Autodesk Inventor part; units mm, degrees
ref_plane "YZ Plane" through (0, 0, 0) normal (1, 0, 0) x (0, 1, 0)
ref_plane "XZ Plane" through (0, 0, 0) normal (0, 1, 0) x (-1, 0, 0)
ref_plane "XY Plane" through (0, 0, 0) normal (0, 0, 1) x (1, 0, 0)
sketch "Sketch_1" plane through (0, 0, 0) normal (0, 0, 1) x (1, 0, 0)
  line L0 (55.5, 0) -> (0, 0)
  line L1 (0, 0) -> (0, 2)
  line L2 (0, 2) -> (0.5, 2.5)
  line L3 (0.5, 2.5) -> (55, 2.5)
  line L4 (55, 2.5) -> (55.5, 2)
  line L5 (55.5, 2) -> (55.5, 0)
  line L6 (55.5, 0) -> (0, 0)
revolve "Revolution1" add sketch "Sketch_1" angle 360 about axis through (55.5, 0, 0) along (1, 0, 0)
sketch "Sketch2" plane through (0, 0, 0) normal (-1, 0, 0) x (0, 0, 1)
  point P0 (0, 0)
hole "Hole1" at (0, 0, 0) direction (1, 0, 0) diameter 2.459 depth 8.2901 tip angle 120 countersink diameter 3 countersink angle 90
sketch "Sketch3" plane through (55.5, 0, 0) normal (1, 0, 0) x (0, 0, -1)
  point P0 (0, 0)
hole "Hole2" at (55.5, 0, 0) direction (-1, 0, 0) diameter 2.459 depth 8.2901 tip angle 120 countersink diameter 3 countersink angle 90
properties part number "SETF5-55.5-M3-N3" material "ステンレス鋼 AISI 304"
Verification items for the finished model (mm, model axes). A direction names the side the tool comes from. Round coordinates to 2 decimals unless told otherwise and drop trailing zeros. Write each loop counter-clockwise with the first axis right and the second up, starting at its lowest first coordinate (ties: lowest second). Pieces come first, ordered by that corner, then holes.
1. Section check A-A on x = 39.5. Enter the section's corners in (y, z), plus the area to 3 significant figures.
2. Access from +Z, -Z, +X, -X, +Y, -Y to the whole of each face (thin tool, end or side, straight path). Record for faces 3 (the cylindrical face through (51.164, 0.748, 0.976)), 4 (the conical face through (9, 0, 0)).
3. Scan lines: L1, parallel to Z at x = 52.5, y = 0; L2, parallel to Z at x = 23, y = -0.2; L3, parallel to X at y = -1.55, z = -1.65. Record each from-to range of solid material in increasing order.
4. Gauge pin test, flat ends, axial feed: P1, Ø1.5, axis at x = 34, z = -1.5, coming from the -Y side; P2, Ø2, axis at y = 0, z = 0, coming from the -X side. Record the tip position at first contact, or that the pin passes through.
5. Draft check along Y on faces 1 (the cylindrical face through (4.336, 0.748, -0.976)), 2 (the cylindrical face through (28.13, -0.54, -2.44)). Enter one of: +Y half, -Y half, draft (parallel to the pull), parting line (faces both ways), or undercut.
Answer:
1. outline: circle Ø5 at (0, 0)
1. area: 19.6 mm2
2. face 3: +X
2. face 4: -X
3. L1: z = -2.5 to -1.23, 1.23 to 2.5
3. L2: z = -2.49 to 2.49
3. L3: x = 0.26 to 55.24
4. P1: stops at y = -2.38
4. P2: stops at x = 8.42
5. face 1: undercut
5. face 2: parting line
